Geometry check sheet. Reference: the model listing, model coordinates, mm. A direction names the side the tool comes from. Round coordinates to 2 decimals unless told otherwise and drop trailing zeros. Write each loop counter-clockwise with the first axis right and the second up, starting at its lowest first coordinate (ties: lowest second). Pieces come first, ordered by that corner, then holes. Notation, with made-up numbers: M -26.75,0 L -15.75,0 A21 ccw -15.75,33 Z; hole C -35,54 d8. An arc over 180 degrees is marked long. Use a Markdown table: item, result.
```python
from build123d import *

# Parameters (mm, degrees)
EXTRUDE_1_DEPTH          = 6
EXTRUDE_1_DEPTH_BACK     = 6
SKETCH_1_R               = 2.5
CUT_EXTRUDE_1_DEPTH      = 3
CUT_EXTRUDE_1_DEPTH_BACK = 3
SKETCH_2_W               = 15
SKETCH_2_H               = 13
CUT_EXTRUDE_2_DEPTH      = 6


with BuildPart() as part:
    # Эскиз1 → Бобышка-Вытянуть1 (new, two sides: drawn at the far end of the back side and taken through both)
    # profile 1 of 9: a face of its own
    with BuildSketch(Plane.XY.offset(-EXTRUDE_1_DEPTH_BACK)):
        with BuildLine():
            Line((5, 15.724185194), (5, 8.660254038))
            ThreePointArc((5, 8.660254038), (8.660254038, 5), (10, 0))
            Line((10, 0), (16.117543831, -3.531965578))
            ThreePointArc((16.117543831, -3.531965578), (16.404107309, -1.776306108), (16.5, 0))
            ThreePointArc((16.5, 0), (13.318220602, 9.740379869), (5, 15.724185194))
        make_face()
    # profile 2 of 9: a face of its own
    with BuildSketch(Plane.XY.offset(-EXTRUDE_1_DEPTH_BACK)):
        with BuildLine():
            Line((-5, 15.724185194), (-5, 8.660254038))
            ThreePointArc((-5, 8.660254038), (0, 10), (5, 8.660254038))
            Line((5, 8.660254038), (5, 15.724185194))
            ThreePointArc((5, 15.724185194), (0, 16.5), (-5, 15.724185194))
        make_face()
    # profile 3 of 9: a face of its own
    with BuildSketch(Plane.XY.offset(-EXTRUDE_1_DEPTH_BACK)):
        with BuildLine():
            ThreePointArc((-10, 0), (-8.660254038, 5), (-5, 8.660254038))
            Line((-5, 8.660254038), (-5, 15.724185194))
            ThreePointArc((-5, 15.724185194), (-14.289419162, 8.25), (-16.117543831, -3.531965578))
            Line((-16.117543831, -3.531965578), (-10, 0))
        make_face()
    # profile 4 of 9: a face of its own
    with BuildSketch(Plane.XY.offset(-EXTRUDE_1_DEPTH_BACK)):
        with BuildLine():
            ThreePointArc((-5, -8.660254038), (-8.660254038, -5), (-10, 0))
            Line((-10, 0), (-16.117543831, -3.531965578))
            ThreePointArc((-16.117543831, -3.531965578), (-14.289419162, -8.25), (-11.117543831, -12.192219616))
            Line((-11.117543831, -12.192219616), (-5, -8.660254038))
        make_face()
    # profile 5 of 9: a face of its own
    with BuildSketch(Plane.XY.offset(-EXTRUDE_1_DEPTH_BACK)):
        with BuildLine():
            ThreePointArc((5, -8.660254038), (0, -10), (-5, -8.660254038))
            Line((-5, -8.660254038), (-11.117543831, -12.192219616))
            ThreePointArc((-11.117543831, -12.192219616), (0, -16.5), (11.117543831, -12.192219616))
            Line((11.117543831, -12.192219616), (5, -8.660254038))
        make_face()
    # profile 6 of 9: a face of its own
    with BuildSketch(Plane.XY.offset(-EXTRUDE_1_DEPTH_BACK)):
        with BuildLine():
            ThreePointArc((10, 0), (8.660254038, -5), (5, -8.660254038))
            Line((5, -8.660254038), (11.117543831, -12.192219616))
            ThreePointArc((11.117543831, -12.192219616), (14.289419162, -8.25), (16.117543831, -3.531965578))
            Line((16.117543831, -3.531965578), (10, 0))
        make_face()
    # profile 7 of 9: a face of its own
    with BuildSketch(Plane.XY.offset(-EXTRUDE_1_DEPTH_BACK)):
        with BuildLine():
            ThreePointArc((16.117543831, -3.531965578), (14.289419162, -8.25), (11.117543831, -12.192219616))
            Line((11.117543831, -12.192219616), (20.016660498, -17.330127019))
            ThreePointArc((20.016660498, -17.330127019), (26.846787517, -15.5), (25.016660498, -8.669872981))
            Line((25.016660498, -8.669872981), (16.117543831, -3.531965578))
        make_face()
        with Locations((22.516660498, -13)):
            Circle(SKETCH_1_R, mode=Mode.SUBTRACT)
    # profile 8 of 9: a face of its own
    with BuildSketch(Plane.XY.offset(-EXTRUDE_1_DEPTH_BACK)):
        with BuildLine():
            ThreePointArc((-11.117543831, -12.192219616), (-14.289419162, -8.25), (-16.117543831, -3.531965578))
            Line((-16.117543831, -3.531965578), (-25.016660498, -8.669872981))
            ThreePointArc((-25.016660498, -8.669872981), (-26.846787517, -15.5), (-20.016660498, -17.330127019))
            Line((-20.016660498, -17.330127019), (-11.117543831, -12.192219616))
        make_face()
        with Locations((-22.516660498, -13)):
            Circle(SKETCH_1_R, mode=Mode.SUBTRACT)
    # profile 9 of 9: a face of its own
    with BuildSketch(Plane.XY.offset(-EXTRUDE_1_DEPTH_BACK)):
        with BuildLine():
            Line((-5, 26), (-5, 15.724185194))
            ThreePointArc((-5, 15.724185194), (0, 16.5), (5, 15.724185194))
            Line((5, 15.724185194), (5, 26))
            ThreePointArc((5, 26), (0, 31), (-5, 26))
        make_face()
        with Locations((0, 26)):
            Circle(SKETCH_1_R, mode=Mode.SUBTRACT)
    extrude(amount=EXTRUDE_1_DEPTH + EXTRUDE_1_DEPTH_BACK)

    # Эскиз2 → Вырез-Вытянуть1 (cut, two sides: drawn at the far end of the back side and taken through both)
    with BuildSketch(Plane.XY.offset(-CUT_EXTRUDE_1_DEPTH_BACK)):
        with Locations((0, 26)):
            Rectangle(SKETCH_2_W, SKETCH_2_H)
    extrude(amount=CUT_EXTRUDE_1_DEPTH + CUT_EXTRUDE_1_DEPTH_BACK, mode=Mode.SUBTRACT)

    # Эскиз3 → Вырез-Вытянуть2 (cut)
    with BuildSketch(Plane.XY.offset(-3)):
        Polygon((-22.212812921, -25.526279442), (-11.820508076, -19.526279442), (-22.820508076, -0.473720558), (-33.212812921, -6.473720558), align=None)
    extrude(amount=CUT_EXTRUDE_2_DEPTH, mode=Mode.SUBTRACT)


solid = part.part
```
Item 1: Mould release check, pull along X, two halves, no side actions. Record for faces 1 (the face through (24.826, -13.958, -0.084)), 2 (the face through (0, 31, 4)), 3 (the face through (-21.363, -15.218, 4.479)), 4 (the face through (-14.2, 8.4, -0.1)): +X half, -X half, draft (parallel to the pull), parting line (faces both ways), or undercut.
Outcome:
| item | result |
|---|---|
| face 1 | undercut |
| face 2 | parting line |
| face 3 | undercut |
| face 4 | -X half |
Item 2: Cross-section at B-B, the plane x = 0. Record the cut outline in (y, z).
Outcome:
| item | result |
|---|---|
| outline | M -16.5,-6 L -10,-6 L -10,6 L -16.5,6 Z; M 10,-6 L 23.5,-6 L 23.5,-3 L 19.5,-3 L 19.5,3 L 23.5,3 L 23.5,6 L 10,6 Z; M 28.5,-6 L 31,-6 L 31,-3 L 28.5,-3 Z; M 28.5,3 L 31,3 L 31,6 L 28.5,6 Z |
Item 3: Cross-section at A-A, the plane z = 1. Record the cut outline in (x, y).
Outcome:
| item | result |
|---|---|
| outline | M -19.82,-5.67 L -14.82,-14.33 L -11.12,-12.19 A16.5 ccw 11.12,-12.19 L 20.02,-17.33 A5 ccw 25.02,-8.67 L 16.12,-3.53 A16.5 ccw 5,15.72 L 5,19.5 L -5,19.5 L -5,15.72 A16.5 ccw -16.12,-3.53 Z; hole C 0,0 d20; hole C 22.52,-13 d5 |
Item 4: Access from +Z, -Z, +X, -X, +Y, -Y to the whole of each face (thin tool, end or side, straight path). Record for faces 5 (the face through (-20, -12, -3)), 6 (the face through (-5, 19, 0)), 7 (the face through (0, 23, 3)).
Outcome:
| item | result |
|---|---|
| face 5 | -X, -Y |
| face 6 | +Z, -Z, -X, +Y |
| face 7 | +X, -X, +Y |
Item 5: Material ranges on line 1 along X through (y, z) = (26, 4.3); line 2 along X through (y, z) = (21, -3.5); line 3 along Y through (x, z) = (3, -2), recorded low to high. Write a range as from..to.
Outcome:
| item | result |
|---|---|
| line 1 | x = -5..-2.5, 2.5..5 |
| line 2 | x = -5..5 |
| line 3 | y = -16.22..-9.54, 9.54..19.5 |
Item 6: Go/stop test with flat-tipped pins: pin 1 (2 mm diameter, centred on y = 11.5, z = -3.5, fed in from +X); pin 2 (5 mm diameter, centred on y = 20.5, z = -2.5, fed in from -X); pin 3 (3 mm diameter, centred on x = 0, z = 1, fed in from +Y). Record where each tip stops, or that it passes through.
Outcome:
| item | result |
|---|---|
| pin 1 | stops at x = 12.73 |
| pin 2 | stops at x = -5 |
| pin 3 | stops at y = 19.5 |
Item 7: Cross-section at C-C, the plane y = -13. Record the cut outline in (x, z), and give its area (3 significant figures).
Outcome:
| item | result |
|---|---|
| outline | M -27.52,-6 L -25.02,-6 L -25.02,-3 L -27.52,-3 Z; M -27.52,3 L -25.02,3 L -25.02,6 L -27.52,6 Z; M -20.02,-6 L -12.52,-6 L -12.52,6 L -20.02,6 L -20.02,3 L -15.59,3 L -15.59,-3 L -20.02,-3 Z; M -10.16,-6 L 10.16,-6 L 10.16,6 L -10.16,6 Z; M 12.52,-6 L 20.02,-6 L 20.02,6 L 12.52,6 Z; M 25.02,-6 L 27.52,-6 L 27.52,6 L 25.02,6 Z |
| area | 442 mm2 |
Item 8: Cross-section at D-D, the plane z = -4.5. Record the cut outline in (x, y), and give its area (3 significant figures).
Outcome:
| item | result |
|---|---|
| outline | M -25.02,-8.67 A5 ccw -20.02,-17.33 L -11.12,-12.19 A16.5 ccw 11.12,-12.19 L 20.02,-17.33 A5 ccw 25.02,-8.67 L 16.12,-3.53 A16.5 ccw 5,15.72 L 5,26 A5 ccw -5,26 L -5,15.72 A16.5 ccw -16.12,-3.53 Z; hole C -22.52,-13 d5; hole C 0,0 d20; hole C 0,26 d5; hole C 22.52,-13 d5 |
| area | 893 mm2 |
